```python
from build123d import *
from build123d.topology import SkipClean

# Parameters (mm, degrees)
EXTRUDE_1_DEPTH          = 1.5
EXTRUDE_2_DEPTH          = 30
EXTRUDE_3_DEPTH          = 1
SKETCH_4_R               = 42
SKETCH_4_R_2             = 40.5
EXTRUDE_4_DEPTH          = 11
SKETCH_5_R               = 44.50000000000001
SKETCH_5_R_2             = 40.5
EXTRUDE_5_DEPTH          = 2
SKETCH_6_R               = 42
SKETCH_6_R_2             = 40.5
EXTRUDE_6_DEPTH          = 6
SKETCH_7_R               = 11
CUT_EXTRUDE_1_DEPTH      = 108.14505354891564
PATTERN_CIRCULAR_1_COUNT = 2
PATTERN_CIRCULAR_1_ANGLE = 90.0000000000002


with BuildPart() as part:
    # Эскиз1 → Бобышка-Вытянуть1 (new body)
    with BuildSketch(Plane(origin=(0, 0, 0), x_dir=(1, 0, 0), z_dir=(0, 1, 0))):
        with BuildLine():
            Line((17.347550259331598, 38.25), (-17.347550259330436, 38.25))
            ThreePointArc((-17.347550259330443, 38.25000000000006), (-29.698484809834387, 29.698484809835605), (-38.24999999999934, 17.34755025933202))
            Line((-38.25, 17.34755025933216), (-38.25, -17.34755025933218))
            ThreePointArc((-38.249999999999325, -17.347550259332046), (-29.698484809834383, -29.698484809835612), (-17.34755025933046, -38.25000000000004))
            Line((-17.347550259330426, -38.25), (17.34755025933157, -38.25))
            ThreePointArc((17.347550259331467, -38.249999999999595), (29.69848480983491, -29.698484809835083), (38.24999999999949, -17.347550259331687))
            Line((38.25, -17.34755025933179), (38.25, 17.347550259331754))
            ThreePointArc((38.2499999999995, 17.347550259331655), (29.69848480983494, 29.69848480983505), (17.347550259331513, 38.249999999999574))
        make_face()
    extrude(amount=EXTRUDE_1_DEPTH)

    # Эскиз2 → Бобышка-Вытянуть2 (add)
    with BuildSketch(Plane(origin=(0, 1.5, 0), x_dir=(1, 0, 0), z_dir=(0, 1, 0))):
        with BuildLine():
            Line((-17.34755025933057, -38.25), (17.34755025933057, -38.25))
            ThreePointArc((17.34755025933057, -38.25), (29.698484809834998, -29.698484809834994), (38.25, -17.347550259330568))
            Line((38.25, -17.347550259330568), (38.25, 17.34755025933057))
            ThreePointArc((38.25, 17.34755025933057), (29.698484809834998, 29.698484809834994), (17.347550259330568, 38.25))
            Line((17.347550259330568, 38.25), (-17.34755025933057, 38.25))
            ThreePointArc((-17.34755025933057, 38.25), (-29.698484809834994, 29.698484809834998), (-38.25, 17.347550259330582))
            Line((-38.25, 17.347550259330582), (-38.25, -17.34755025933057))
            ThreePointArc((-38.25, -17.34755025933057), (-29.698484809834994, -29.698484809834998), (-17.34755025933057, -38.25))
        make_face()
        with BuildLine():
            Line((-17.020208576865333, -36.75), (17.020208576865333, -36.75))
            ThreePointArc((17.020208576865333, -36.75), (28.637824638055175, -28.63782463805517), (36.75, -17.020208576865333))
            Line((36.75, -17.020208576865333), (36.75, 17.020208576865333))
            ThreePointArc((36.75, 17.020208576865333), (28.637824638055175, 28.63782463805517), (17.020208576865333, 36.75))
            Line((17.020208576865333, 36.75), (-17.020208576865333, 36.75))
            ThreePointArc((-17.020208576865333, 36.75), (-28.63782463805517, 28.637824638055175), (-36.75, 17.020208576865333))
            Line((-36.75, 17.020208576865333), (-36.75, -17.020208576865333))
            ThreePointArc((-36.75, -17.020208576865333), (-28.63782463805517, -28.637824638055175), (-17.020208576865333, -36.75))
        make_face(mode=Mode.SUBTRACT)
    extrude(amount=EXTRUDE_2_DEPTH)

    # Эскиз3 → Бобышка-Вытянуть3 (add)
    with BuildSketch(Plane(origin=(0, 31.5, 0), x_dir=(1, 0, 0), z_dir=(0, 1, 0))):
        with BuildLine():
            Line((-38.25, -13.31117951197428), (-38.249999999999986, 13.311179511974292))
            ThreePointArc((-38.24999999999994, 13.311179511974292), (-40.5, 4.96e-15), (-38.24999999999996, -13.311179511974263))
        make_face()
        with BuildLine():
            ThreePointArc((-36.74999999999999, 17.02020857686534), (-37.545828318883174, 15.184227864759881), (-38.24999999999994, 13.311179511974292))
            Line((-38.249999999999986, 13.311179511974292), (-38.25, -13.31117951197428))
            ThreePointArc((-38.24999999999996, -13.311179511974263), (-37.54582831888318, -15.184227864759869), (-36.75, -17.02020857686533))
            Line((-36.75, -17.020208576865333), (-36.75, 17.02020857686534))
        make_face()
        with BuildLine():
            ThreePointArc((38.25, -17.347550259330568), (41.05179655021202, -8.874119674649448), (42, -1.029e-14))
            ThreePointArc((42, 0), (41.051796550212025, 8.874119674649428), (38.24999999999999, 17.347550259330575))
            Line((38.25, 17.347550259330568), (38.25, 13.311179511973094))
            ThreePointArc((38.25000000000035, 13.311179511973151), (39.933538535922494, 6.749999999999486), (40.5, 0))
            ThreePointArc((40.5, -9.92e-15), (39.933538535922494, -6.749999999999494), (38.25000000000033, -13.311179511973192))
            Line((38.25, -13.311179511973124), (38.25, -17.347550259330568))
        make_face()
        with BuildLine():
            ThreePointArc((40.5, 0), (39.933538535922494, 6.749999999999486), (38.25000000000035, 13.311179511973151))
            Line((38.25, 13.311179511973094), (38.25, -13.311179511973124))
            ThreePointArc((38.25000000000033, -13.311179511973192), (39.933538535922494, -6.749999999999494), (40.5, -9.92e-15))
        make_face()
        with BuildLine():
            Line((38.25, -13.311179511973124), (38.25, 13.311179511973094))
            ThreePointArc((38.25000000000035, 13.311179511973151), (37.5458283188834, 15.184227864759325), (36.75, 17.020208576865333))
            Line((36.75, 17.020208576865333), (36.75, -17.020208576865333))
            ThreePointArc((36.74999999999999, -17.020208576865343), (37.54582831888339, -15.18422786475935), (38.25000000000033, -13.311179511973192))
        make_face()
        with BuildLine():
            ThreePointArc((17.02020857686533, 36.75), (15.18422786475986, 37.54582831888318), (13.311179511974236, 38.249999999999964))
            Line((13.311179511974245, 38.25000000000001), (-13.311179511974242, 38.25))
            ThreePointArc((-13.311179511974233, 38.249999999999964), (-15.184227864759857, 37.54582831888318), (-17.020208576865333, 36.75))
            Line((-17.020208576865333, 36.75), (17.020208576865326, 36.75000000000001))
        make_face()
        with BuildLine():
            Line((-13.311179511974242, 38.25), (13.311179511974245, 38.25000000000001))
            ThreePointArc((13.311179511974236, 38.249999999999964), (2.48e-15, 40.5), (-13.311179511974233, 38.249999999999964))
        make_face()
        with BuildLine():
            Line((13.311179511974245, 38.25000000000001), (17.347550259330564, 38.25000000000001))
            ThreePointArc((17.34755025933056, 38.25000000000001), (-6.75e-15, 42), (-17.34755025933057, 38.25))
            Line((-17.34755025933057, 38.25), (-13.311179511974242, 38.25))
            ThreePointArc((-13.311179511974233, 38.249999999999964), (2.48e-15, 40.5), (13.311179511974236, 38.249999999999964))
        make_face()
        with BuildLine():
            ThreePointArc((-17.347550259330596, -38.249999999999986), (-7.72e-15, -42), (17.347550259330582, -38.24999999999999))
            Line((17.34755025933057, -38.25), (13.311179511974295, -38.25))
            ThreePointArc((13.311179511974295, -38.24999999999994), (2.853e-14, -40.5), (-13.311179511974242, -38.249999999999964))
            Line((-13.311179511974242, -38.25), (-17.34755025933057, -38.25))
        make_face()
        with BuildLine():
            ThreePointArc((-13.311179511974242, -38.249999999999964), (2.853e-14, -40.5), (13.311179511974295, -38.24999999999994))
            Line((13.311179511974295, -38.25), (-13.311179511974242, -38.25))
        make_face()
        with BuildLine():
            Line((-13.311179511974242, -38.25), (13.311179511974295, -38.25))
            ThreePointArc((13.311179511974295, -38.24999999999994), (15.184227864759867, -37.54582831888318), (17.02020857686533, -36.75))
            Line((17.020208576865333, -36.75), (-17.020208576865333, -36.75))
            ThreePointArc((-17.020208576865343, -36.74999999999999), (-15.18422786475985, -37.54582831888319), (-13.311179511974242, -38.249999999999964))
        make_face()
        with BuildLine():
            ThreePointArc((-38.25, -17.347550259330568), (-29.698484809835, -29.698484809834994), (-17.347550259330596, -38.249999999999986))
            Line((-17.34755025933057, -38.25), (-13.311179511974242, -38.25))
            ThreePointArc((-13.311179511974242, -38.249999999999964), (-15.18422786475985, -37.54582831888319), (-17.020208576865343, -36.74999999999999))
            ThreePointArc((-17.020208576865343, -36.74999999999999), (-28.637824638055182, -28.63782463805517), (-36.75, -17.02020857686533))
            ThreePointArc((-36.75, -17.02020857686533), (-37.54582831888318, -15.184227864759869), (-38.24999999999996, -13.311179511974263))
            Line((-38.25, -13.31117951197428), (-38.25, -17.34755025933057))
        make_face()
        with BuildLine():
            ThreePointArc((17.347550259330582, -38.24999999999999), (29.698484809835016, -29.698484809834973), (38.25, -17.347550259330568))
            Line((38.25, -17.347550259330568), (38.25, -13.311179511973124))
            ThreePointArc((38.25000000000033, -13.311179511973192), (37.54582831888339, -15.18422786475935), (36.74999999999999, -17.020208576865343))
            ThreePointArc((36.74999999999999, -17.020208576865343), (28.637824638055168, -28.637824638055182), (17.02020857686533, -36.75))
            ThreePointArc((17.02020857686533, -36.75), (15.184227864759867, -37.54582831888318), (13.311179511974295, -38.24999999999994))
            Line((13.311179511974295, -38.25), (17.34755025933057, -38.25))
        make_face()
        with BuildLine():
            Line((38.25, 13.311179511973094), (38.25, 17.347550259330568))
            ThreePointArc((38.24999999999999, 17.347550259330575), (29.698484809834987, 29.698484809835), (17.34755025933056, 38.25000000000001))
            Line((17.347550259330564, 38.25000000000001), (13.311179511974245, 38.25000000000001))
            ThreePointArc((13.311179511974236, 38.249999999999964), (15.18422786475986, 37.54582831888318), (17.02020857686533, 36.75))
            ThreePointArc((17.02020857686533, 36.75), (28.637824638055175, 28.63782463805517), (36.75, 17.020208576865333))
            ThreePointArc((36.75, 17.020208576865333), (37.5458283188834, 15.184227864759325), (38.25000000000035, 13.311179511973151))
        make_face()
        with BuildLine():
            Line((-13.311179511974242, 38.25), (-17.34755025933057, 38.25))
            ThreePointArc((-17.34755025933057, 38.25), (-29.69848480983498, 29.698484809835012), (-38.24999999999998, 17.347550259330614))
            Line((-38.249999999999986, 17.3475502593306), (-38.249999999999986, 13.311179511974292))
            ThreePointArc((-38.24999999999994, 13.311179511974292), (-37.545828318883174, 15.184227864759881), (-36.74999999999999, 17.02020857686534))
            ThreePointArc((-36.74999999999999, 17.02020857686534), (-28.63782463805517, 28.637824638055175), (-17.020208576865333, 36.75))
            ThreePointArc((-17.020208576865333, 36.75), (-15.184227864759857, 37.54582831888318), (-13.311179511974233, 38.249999999999964))
        make_face()
        with BuildLine():
            Line((-38.249999999999986, 13.311179511974292), (-38.249999999999986, 17.3475502593306))
            ThreePointArc((-38.24999999999998, 17.347550259330614), (-42, 2.38e-14), (-38.25, -17.347550259330568))
            Line((-38.25, -17.34755025933057), (-38.25, -13.31117951197428))
            ThreePointArc((-38.24999999999996, -13.311179511974263), (-40.5, 4.96e-15), (-38.24999999999994, 13.311179511974292))
        make_face()
    extrude(amount=EXTRUDE_3_DEPTH)

    # Эскиз4 → Бобышка-Вытянуть4 (add)
    with SkipClean():  # the faces are left unmerged after this step: merging them gives an invalid solid
        with BuildSketch(Plane(origin=(0, 32.5, 0), x_dir=(1, 0, 0), z_dir=(0, 1, 0))):
            with Locations(Location((0, 0, 0), (0, 0, 65.604247888))):
                Circle(SKETCH_4_R)
            with Locations(Location((0, 0, 0), (0, 0, 65.14949766))):
                Circle(SKETCH_4_R_2, mode=Mode.SUBTRACT)
        extrude(amount=EXTRUDE_4_DEPTH)

    # Эскиз5 → Бобышка-Вытянуть5 (add)
    with BuildSketch(Plane(origin=(0, 43.5, 0), x_dir=(1, 0, 0), z_dir=(0, 1, 0))):
        with Locations(Location((0, 0, 0), (0, 0, 270))):
            Circle(SKETCH_5_R)
        with Locations(Location((0, 0, 0), (0, 0, 65.14949766))):
            Circle(SKETCH_5_R_2, mode=Mode.SUBTRACT)
    extrude(amount=EXTRUDE_5_DEPTH)

    # Эскиз6 → Бобышка-Вытянуть6 (add)
    with BuildSketch(Plane(origin=(0, 45.5, 0), x_dir=(1, 0, 0), z_dir=(0, 1, 0))):
        with Locations(Location((0, 0, 0), (0, 0, 65.604247888))):
            Circle(SKETCH_6_R)
        with Locations(Location((0, 0, 0), (0, 0, 65.14949766))):
            Circle(SKETCH_6_R_2, mode=Mode.SUBTRACT)
    extrude(amount=EXTRUDE_6_DEPTH)

    # Эскиз7 → Вырез-Вытянуть1 (cut, through all)
    with BuildSketch(Plane(origin=(38.25, 0, 0), x_dir=(0, 0, -1), z_dir=(1, 0, 0))):
        with Locations((0, 16)):
            Circle(SKETCH_7_R)
    cut_extrude_1 = extrude(amount=-CUT_EXTRUDE_1_DEPTH, mode=Mode.SUBTRACT)

    # Круговой массив1: Вырез-Вытянуть1 ×2 about axis
    pattern_circular_1_axis = Axis((0, 0, 0), (0, -1, 0))
    for i in range(1, PATTERN_CIRCULAR_1_COUNT):
        add(cut_extrude_1.rotate(pattern_circular_1_axis, i * PATTERN_CIRCULAR_1_ANGLE / (PATTERN_CIRCULAR_1_COUNT - 1)), mode=Mode.SUBTRACT)


solid = part.part
```
Geometry: final body of the model. Coordinates: model frame, mm. A direction names the side the tool comes from. Round coordinates to 2 decimals unless told otherwise and drop trailing zeros. Order: outer loops, then holes, each group sorted by start corner. A loop starts at its lowest first (then second) coordinate and runs counter-clockwise, first axis right, second up. Notation, with made-up numbers: (-26.5, -31.5) -> (23.5, -31.5) arc R27 ccw to (23.5, -15.5) -> close; hole circle Ø8 at (-39, 50). An arc over 180 degrees is marked (long way). Use CSV: the item, a comma, the result in double quotes. Start each with the question number.
1) Section D-D (y = 41). Return the cut outline in (x, z).
2) Section A-A (z = 0). State how many separate pieces and enclosed holes the cut face has, and give its area (3 significant figures).
3) Draft query along Y for faces 5 (the face through (0, 32.5, -38)), 6 (the face through (37.51, 5.26, 2.38)), 7 (the face through (38.25, 5, 4)). Return one class per face: +Y half, -Y half, draft (parallel to the pull), parting line (faces both ways), or undercut.
4) Set-up query: faces 1 (the face through (5.057, 48.458, -41.694)), 2 (the face through (-38.25, 5, 4)), 3 (the face through (40, 31.5, 0)), 4 (the face through (0, 31.5, -40)). Return all of +Z, -Z, +X, -X, +Y, -Y with unobstructed straight access to the full face (end or side cutting, diameter ignored); none if empty.
5) First-contact query: pin 1 Ø3 at (y, z) = (31.5, -2) entering from +X; pin 2 Ø15.5 at (y, z) = (18.5, 4.5) entering from +X; pin 3 Ø1.5 at (x, z) = (-4.5, -15.5) entering from +Y. Flat tips, straight axial feed; report the tip coordinate or a pass-through.
6) Material intervals for line 1 along Y through (x, z) = (0, 37); line 2 along X through (y, z) = (3, -8.5); line 3 along Z through (x, y) = (0, 47.75), sorted ascending. Write a range as from..to.
Returned:
1,outline,"circle Ø84 at (0, 0); hole circle Ø81 at (0, 0)"
2,separate pieces,"3"
2,enclosed holes,"0"
2,area,"216 mm²"
3,face 5,"+Y half"
3,face 6,"undercut"
3,face 7,"draft"
4,face 1,"+Y"
4,face 2,"+Z, -Z, -X, -Y"
4,face 3,"+Z, -Z, +X, -Y"
4,face 4,"-Z, +X, -X, -Y"
5,pin 1,"stops at x = 42"
5,pin 2,"stops at x = 38.25"
5,pin 3,"stops at y = 1.5"
6,line 1,"y = 0..5, 27..32.5"
6,line 2,"x = -38.25..-36.75, 36.75..38.25"
6,line 3,"z = -42..-40.5, 40.5..42"
